The model under review builds one solid part; all positions refer to its coordinate system, in mm. A direction names the side the tool comes from. Give positions to 0.01 mm unless a question says otherwise; leave off trailing zeros. Order: outer loops, then holes, each group sorted by start corner. A loop starts at its lowest first (then second) coordinate and runs counter-clockwise, first axis right, second up. Notation, with made-up numbers: (85.5, 37.25) -> (96.5, 37.25) arc R23 ccw to (96.5, 48.25) -> close; hole circle Ø6 at (72.25, 46). An arc over 180 degrees is marked (long way). Answer as a JSON object with one key per item and string values. Group by question number.
Autodesk Inventor part; units mm, degrees
ref_plane "YZ Plane" through (0, 0, 0) normal (1, 0, 0) x (0, 1, 0)
ref_plane "XZ Plane" through (0, 0, 0) normal (0, 1, 0) x (-1, 0, 0)
ref_plane "XY Plane" through (0, 0, 0) normal (0, 0, 1) x (1, 0, 0)
sketch "スケッチ1" plane through (0, 0, 0) normal (0, 0, 1) x (1, 0, 0)
  line L0 (0, 0) -> (0, 2.6709) construction
  circle A0 centre (-18.5, 0) radius 1.3
  circle A1 centre (18.5, 0) radius 1.3
  circle A2 centre (-18.5, 0) radius 3
  circle A3 centre (18.5, 0) radius 3
  line L1 (-18.5, 3) -> (18.5, 3)
  line L2 (-18.5, -3) -> (18.5, -3)
  line L3 (-15.25, 6) -> (15.25, 6)
  line L4 (15.25, 6) -> (15.25, -15)
  line L5 (15.25, -15) -> (-15.25, -15)
  line L6 (-15.25, -15) -> (-15.25, 6)
  point P0 (-18.5, 3)
  point P1 (15.25, -3)
  point P2 (-15.25, -3)
  point P3 (-15.25, 3)
  point P4 (15.25, 3)
  point P5 (0, 6)
  point P6 (0, 3)
  dimension "d0" = 2.6
  dimension "d1" = 18.5
  dimension "d2" = 6
  dimension "d3" = 6
  dimension "d6" = 3
  dimension "d7" = 12
  dimension "d9" = 30.5
extrude "押し出し1" add sketch "スケッチ1" along normal blind 3
fillet "フィレット1" radius 2 6 edges at (-15.25, 3, 1.5) (-15.25, -3, 1.5) (15.25, 3, 1.5) (15.25, -3, 1.5) (-15.25, 6, 1.5) (15.25, 6, 1.5)
sketch "スケッチ4" plane through (0, 0, 0) normal (0, 0, -1) x (-1, 0, 0)
  line L0 (-12.25, 4) -> (12.25, 4)
  line L1 (12.25, 4) -> (12.25, -13)
  line L2 (12.25, -13) -> (-12.25, -13)
  line L3 (-12.25, -13) -> (-12.25, 4)
  line L4 (15.25, -15) -> (-15.25, -15)
  line L5 (-13.377, 6) -> (13.377, 6)
  line L6 (-15.25, -15) -> (-15.25, -5)
  line L7 (15.25, -5) -> (15.25, -15)
  point P0 (0, 0)
  dimension "d27" = 2
  dimension "d28" = 2
  dimension "d32" = 3
  dimension "d33" = 3
extrude "押し出し3" cut sketch "スケッチ4" against normal through all
fillet "フィレット2" radius 2 4 edges at (12.25, 4, 1.5) (-12.25, 4, 1.5) (12.25, -13, 1.5) (-12.25, -13, 1.5)
sketch "スケッチ2" plane through (15.25, -15, 3) normal (1, 0, 0) x (0, 0, -1)
  line L0 (3, 0) -> (0, 0)
  point P0 (3, 15)
  point P1 (1.5, 3)
  point P2 (1.5, 8)
  point P3 (1.5, 0)
  dimension "d10" = 3
  dimension "d11" = 5
hole "穴1" at (15.25, -12, 1.5) at (15.25, -7, 1.5) direction (-1, 0, 0) diameter 1.567 end through all
sketch "スケッチ3" plane through (0, 0, 3) normal (0, 0, 1) x (1, 0, 0)
  line L0 (-15.25, -12.7835) -> (-15.25, -11.2165) construction
  line L1 (-15.25, -7.7835) -> (-15.25, -6.2165) construction
  line L2 (15.25, -11.2165) -> (15.25, -12.7835) construction
  line L3 (15.25, -6.2165) -> (15.25, -7.7835) construction
  circle A0 centre (-16.25, -12) radius 1.1
  circle A1 centre (-16.25, -7) radius 1.1
  line L4 (-15.25, -15) -> (15.25, -15) construction
  line L5 (0, -15) -> (0, 6) construction
  line L6 (13.377, 6) -> (-13.377, 6) construction
  line L7 (15.25, -12.7835) -> (15.25, -11.2165) construction
  line L8 (15.25, -7.7835) -> (15.25, -6.2165) construction
  circle A2 centre (16.25, -12) radius 1.1
  circle A3 centre (16.25, -7) radius 1.1
  point P0 (0, 0)
  point P1 (-15.25, -12)
  point P2 (-15.25, -7)
  point P3 (15.25, -12)
  point P4 (15.25, -7)
  dimension "d19" = 2.2
  dimension "d20" = 2.2
  dimension "d21" = 1
  dimension "d22" = 1
extrude "押し出し2" cut sketch "スケッチ3" against normal through all
properties part number "ude_sensor" material "アルミニウム 2014-T4"
1. Draft analysis for pull direction X (two halves, no side actions). For faces 4 (the cylindrical face through (-15.15, -12.01, 0.34)), 5 (the cylindrical face through (-19.8, -0.06, 1.48)), 6 (the cylindrical face through (15.85, -3.57, 1.52)), 7 (the cylindrical face through (-13.771, -6.305, 1.138)), state which applies: pulls with the +X half, pulls with the -X half, needs draft (parallel to the pull), parting line crosses it, or undercut.
2. For pin 1 (0.9 mm diameter, centred on y = -6.5, z = 2, fed in from +X); pin 2 (1.5 mm diameter, centred on y = -1.5, z = 1.5, fed in from -X); pin 3 (1 mm diameter, centred on x = -17.5, z = 1.5, fed in from +Y), all flat-tipped, find the tip position at first contact; note any pin that passes through.
3. Take a section at D-D on z = 1.25. State how many separate pieces and enclosed holes the cut face has, plus the area to 3 significant figures.
4. Machinability: for faces 1 (the flat face through (15.25, -9, 1)), 2 (the cylindrical face through (-13.69, -12.66, 1.08)), 3 (the flat face through (0, -13, 1)), which of the approach directions +Z, -Z, +X, -X, +Y, -Y give a long, thin tool a straight path to every point of the face, cutting with its end or side? Answer none if there is none.
5. For probe 1 along Y at (x, z) = (-12.5, 1.5); probe 2 along X at (y, z) = (-9.25, 0.95); probe 3 along Y at (x, z) = (-9.5, 1.9), list the stretches that pass through material, from the lowest coordinate up. Write a range as [from, to].
6. Take a section at A-A on x = -5. Give the boundary of the cut face in (y, z), plus the area to 3 significant figures.
7. Take a section at C-C on y = 0. Give the boundary of the cut face in (x, z).
8. Take a section at B-B on y = -9.75. Give the boundary of the cut face in (x, z), plus the area to 3 significant figures.
Checks:
{
 "1": {"face 4": "pulls with the -X half", "face 5": "undercut", "face 6": "pulls with the +X half", "face 7": "needs draft"},
 "2": {"pin 1": "stops at x = 15.25", "pin 2": "stops at x = -21.4", "pin 3": "stops at y = 3.02"},
 "3": {"separate pieces": "4", "enclosed holes": "2", "area": "267 mm2"},
 "4": {"face 1": "+Z, -Z, +X, -Y", "face 2": "+X, -X", "face 3": "+Z, -Z"},
 "5": {"probe 1": "y = [-15, -12.78], [-11.22, -7.78], [-6.22, 6]", "probe 2": "x = [-15.25, -12.25], [12.25, 15.25]", "probe 3": "y = [-15, -13], [4, 6]"},
 "6": {"outline": "(-15, 0) -> (-13, 0) -> (-13, 3) -> (-15, 3) -> close; (4, 0) -> (6, 0) -> (6, 3) -> (4, 3) -> close", "area": "12.0 mm2"},
 "7": {"outline": "(-21.5, 0) -> (-19.8, 0) -> (-19.8, 3) -> (-21.5, 3) -> close; (-17.2, 0) -> (-12.25, 0) -> (-12.25, 3) -> (-17.2, 3) -> close; (12.25, 0) -> (17.2, 0) -> (17.2, 3) -> (12.25, 3) -> close; (19.8, 0) -> (21.5, 0) -> (21.5, 3) -> (19.8, 3) -> close"},
 "8": {"outline": "(-15.25, 0) -> (-12.25, 0) -> (-12.25, 3) -> (-15.25, 3) -> close; (12.25, 0) -> (15.25, 0) -> (15.25, 3) -> (12.25, 3) -> close", "area": "18.0 mm2"}
}
